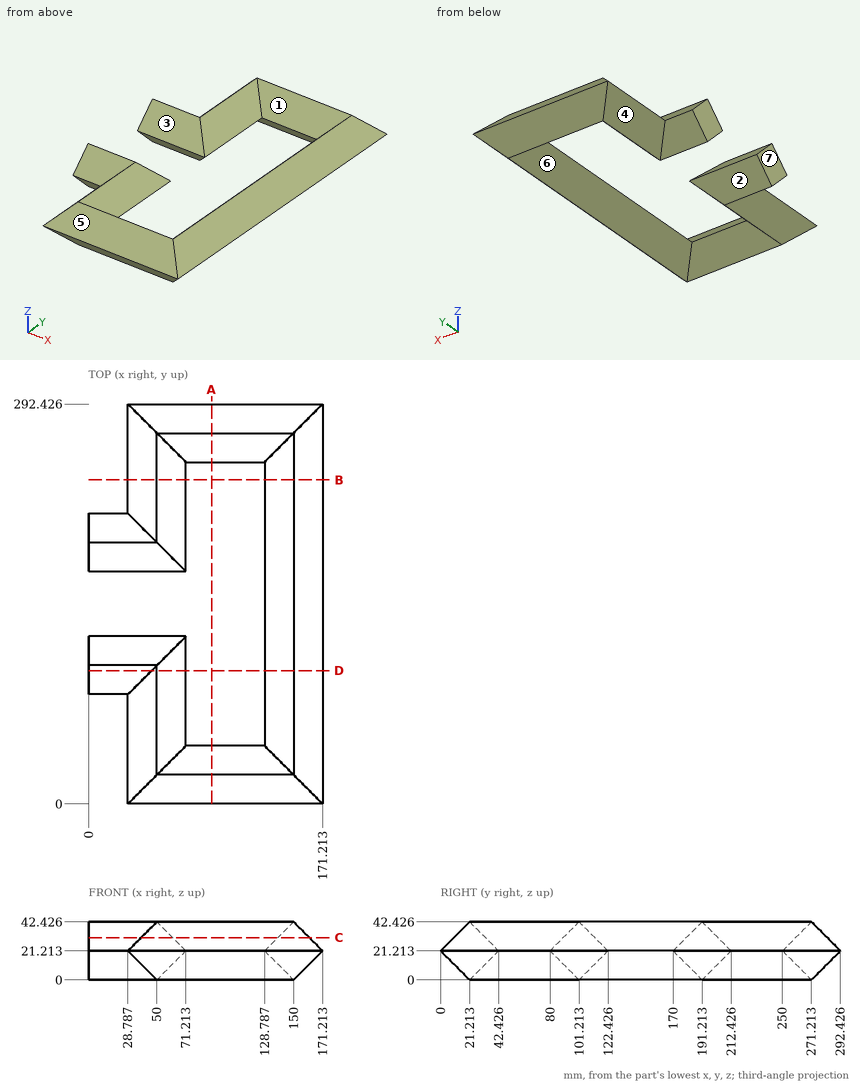
Part print with two shaded views. Sizes in mm from the minimum x, y, z corner. A direction names the side the tool comes from. Coordinates: 2 decimals unless noted, no trailing zeros. Write each loop counter-clockwise with the first axis right and the second up, starting at its lowest first coordinate (ties: lowest second). Pieces come first, ordered by that corner, then holes.
(1) Drill centre lines: line 1 (Y direction, x = 15, z = 26.5) (1 decimal); line 2 (X direction, y = 181, z = 29.5) (1 decimal); line 3 (Y direction, x = 107, z = 4) (1 decimal). Where is each one in solid material? Low to high.
(2) Cut at D-D on y = 97.5. List the corners of the cut face in (x, z).
(3) Pin check, flat tips, straight feed: pin 1 Ø3 at (y, z) = (110.5, 6) entering from +X; pin 2 Ø8 at (y, z) = (110.5, 10.5) entering from +X; pin 3 Ø1.5 at (x, z) = (87.5, 14) entering from -Y. Stop position of each tip, or through.
(4) Cut at A-A on x = 90. List the corners of the cut face in (y, z), and give its area (3 significant figures).
(5) 3-axis set-ups, long thin cutter, end or side, ignore diameter. For the marked faces 1, 2, 3 and 4: which of +Z, -Z, +X, -X, +Y, -Y reach the whole face in a straight line?
(6) Cut at B-B on y = 237. List the corners of the cut face in (x, z), and give its area (3 significant figures).
(7) Cut at C-C on z = 31. List the corners of the cut face in (x, y), and give its area (3 significant figures).
(8) Mould opens along Y. For the marked faces 5, 6 and 7 say: pulls with the +Y half, pulls with the -Y half, needs draft (parallel to the pull), parting line crosses it, or undercut.
Working result:
1. line 1: y = 85.3 to 117.1, 175.3 to 207.1
1. line 2: x = 0 to 62.9, 137.1 to 162.9
1. line 3: y = 17.2 to 25.2, 267.2 to 275.2
2. outline: (0, 3.71) - (46.29, 3.71) - (50, 0) - (71.21, 21.21) - (50, 42.43) - (46.29, 38.71) - (0, 38.71) - close; (128.79, 21.21) - (150, 0) - (171.21, 21.21) - (150, 42.43) - close
3. pin 1: stops at x = 157.5
3. pin 2: stops at x = 164.5
3. pin 3: stops at y = 6.46
4. outline: (0, 21.21) - (21.21, 0) - (42.43, 21.21) - (21.21, 42.43) - close; (250, 21.21) - (271.21, 0) - (292.43, 21.21) - (271.21, 42.43) - close
4. area: 1,800 mm2
5. face 1: +Z
5. face 2: -Z, -X
5. face 3: +Z, -X
5. face 4: -Z, -X, +Y
6. outline: (28.79, 21.21) - (50, 0) - (71.21, 21.21) - (50, 42.43) - close; (128.79, 21.21) - (150, 0) - (171.21, 21.21) - (150, 42.43) - close
6. area: 1,800 mm2
7. outline: (0, 89.79) - (38.57, 89.79) - (38.57, 9.79) - (161.43, 9.79) - (161.43, 282.64) - (38.57, 282.64) - (38.57, 202.64) - (0, 202.64) - (0, 179.79) - (61.43, 179.79) - (61.43, 259.79) - (138.57, 259.79) - (138.57, 32.64) - (61.43, 32.64) - (61.43, 112.64) - (0, 112.64) - close
7. area: 16,200 mm2
8. face 5: pulls with the -Y half
8. face 6: undercut
8. face 7: needs draft
